Here's how the part is built. I have some questions about the finished solid (model axes, mm). Coordinates: 2 decimals unless noted, no trailing zeros.
(1) Please list where these lines run through material, in increasing order: probe 1 along Y at (x, z) = (-50, 1.7); probe 2 along X at (y, z) = (3.5, 1.65); probe 3 along X at (y, z) = (-12.5, 2.35).
(2) For pin 1 Ø1.8 at (x, y) = (-76.46, -74.27) entering from -Z, with a flat end and sliding along its axis, tell me the tip position at first contact or that it passes through.
(3) Imagine slicing it at A-A, the plane z = 0.75. State how many separate pieces and enclosed holes the cut face has, plus the area to 3 significant figures.
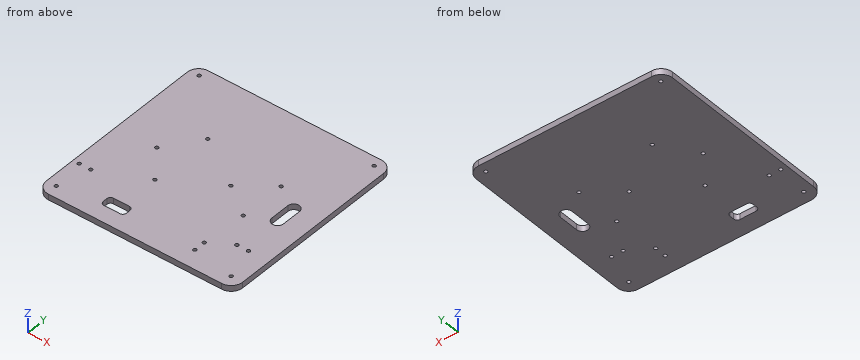
```python
from build123d import *

# Parameters (mm, degrees)
SKETCH1_R           = 1.5
BOSS_EXTRUDE1_DEPTH = 5


with BuildPart() as part:
    # Sketch1 → Boss-Extrude1 (new body)
    with BuildSketch(Plane.XY):
        with BuildLine():
            Line((-75, -84.27), (75, -84.27))
            ThreePointArc((75, -84.27), (82.071067812, -81.341067812), (85, -74.27))
            Line((85, -74.27), (85, 75))
            ThreePointArc((85, 75), (82.071067812, 82.071067812), (75, 85))
            Line((75, 85), (-75, 85))
            ThreePointArc((-75, 85), (-82.071067812, 82.071067812), (-85, 75))
            Line((-85, 75), (-85, -74.27))
            ThreePointArc((-85, -74.27), (-82.071067812, -81.341067812), (-75, -84.27))
        make_face()
        with Locations((-50, 0)):
            Circle(SKETCH1_R, mode=Mode.SUBTRACT)
        with Locations((14, 0)):
            Circle(SKETCH1_R, mode=Mode.SUBTRACT)
        with Locations((56.997765234, -46.145194914)):
            Circle(SKETCH1_R, mode=Mode.SUBTRACT)
        with Locations((66.997765234, -46.145194914)):
            Circle(SKETCH1_R, mode=Mode.SUBTRACT)
        with Locations((-79.533394359, -46.145194914)):
            Circle(SKETCH1_R, mode=Mode.SUBTRACT)
        with Locations((-69.533394359, -46.145194914)):
            Circle(SKETCH1_R, mode=Mode.SUBTRACT)
        with Locations((38.452124501, -68)):
            Circle(SKETCH1_R, mode=Mode.SUBTRACT)
        with Locations((38.452124501, -58)):
            Circle(SKETCH1_R, mode=Mode.SUBTRACT)
        with Locations((75, -74.271781408)):
            Circle(SKETCH1_R, mode=Mode.SUBTRACT)
        with Locations((-76.456437184, -74.271781408)):
            Circle(SKETCH1_R, mode=Mode.SUBTRACT)
        with Locations((-76.456437184, 77.184655776)):
            Circle(SKETCH1_R, mode=Mode.SUBTRACT)
        with Locations((75, 77.184655776)):
            Circle(SKETCH1_R, mode=Mode.SUBTRACT)
        with Locations((40.5412515, 20.733071637)):
            Circle(SKETCH1_R, mode=Mode.SUBTRACT)
        with Locations((-29.453201544, -27.275016672)):
            Circle(SKETCH1_R, mode=Mode.SUBTRACT)
        with Locations((40.545873573, -19.266928096)):
            Circle(SKETCH1_R, mode=Mode.SUBTRACT)
        with Locations((-29.459672448, 28.724982955)):
            Circle(SKETCH1_R, mode=Mode.SUBTRACT)
        with BuildLine():
            Line((-38.703750493, -60), (-24.703750493, -60))
            ThreePointArc((-24.703750493, -60), (-22.58243015, -60.878679656), (-21.703750493, -63))
            Line((-21.703750493, -63), (-21.703750493, -67))
            ThreePointArc((-21.703750493, -67), (-22.58243015, -69.121320344), (-24.703750493, -70))
            Line((-24.703750493, -70), (-38.703750493, -70))
            ThreePointArc((-38.703750493, -70), (-40.825070837, -69.121320344), (-41.703750493, -67))
            Line((-41.703750493, -67), (-41.703750493, -63))
            ThreePointArc((-41.703750493, -63), (-40.825070837, -60.878679656), (-38.703750493, -60))
        make_face(mode=Mode.SUBTRACT)
        with BuildLine():
            Line((66.997765234, 7.870773212), (66.997765234, -9.129226788))
            ThreePointArc((66.997765234, -9.129226788), (61.997765234, -14.129226788), (56.997765234, -9.129226788))
            Line((56.997765234, -9.129226788), (56.997765234, 7.870773212))
            ThreePointArc((56.997765234, 7.870773212), (61.997765234, 12.870773212), (66.997765234, 7.870773212))
        make_face(mode=Mode.SUBTRACT)
    extrude(amount=BOSS_EXTRUDE1_DEPTH)


solid = part.part
```
Recorded:
1. probe 1: y = -84.27 to -1.5, 1.5 to 85
1. probe 2: x = -85 to 57, 67 to 85
1. probe 3: x = -85 to 58.3, 65.69 to 85
2. pin 1: passes through
3. separate pieces: 1
3. enclosed holes: 18
3. area: 28,100 mm2
